Geometry: final body of the model. Coordinates: model frame, mm. A direction names the side the tool comes from. Give positions to 0.01 mm unless a question says otherwise; leave off trailing zeros. Loops run counter-clockwise (first coordinate to the right, second up) from the corner with the lowest first, then second, coordinate; pieces in that order, holes last.
from build123d import *

# Parameters (mm, degrees)
BOSS_EXTRUDE1_DEPTH      = 7
BOSS_EXTRUDE1_DEPTH_BACK = 7
BOSS_EXTRUDE2_DEPTH      = 7
BOSS_EXTRUDE3_DEPTH      = 7


with BuildPart() as part:
    # Sketch1 → Boss-Extrude1 (new, two sides: drawn at the far end of the back side and taken through both)
    with BuildSketch(Plane.XY.offset(-BOSS_EXTRUDE1_DEPTH_BACK)):
        with BuildLine():
            Line((-17.458418155, -11.36484808), (2.465475807, -9.621733225))
            ThreePointArc((2.465475807, -9.621733225), (6.955793602, -11.676837129), (7.491085956, -16.585998774))
            Line((7.491085956, -16.585998774), (-3.072780906, -41.033415882))
            ThreePointArc((-3.072780906, -41.033415882), (-2.24972743, -50.492456592), (6.106881965, -55))
            Line((6.106881965, -55), (21.106881965, -55))
            Line((21.106881965, -55), (21.106881965, -58))
            Line((21.106881965, -58), (6.106881965, -58))
            ThreePointArc((6.106881965, -58), (-3.921049309, -52.59094791), (-4.908713481, -41.240099059))
            Line((-4.908713481, -41.240099059), (5.655153382, -16.79268195))
            ThreePointArc((5.655153382, -16.79268195), (5.333977969, -13.847184963), (2.639787292, -12.614122621))
            Line((2.639787292, -12.614122621), (-17.197282581, -14.349641352))
            Line((-17.197282581, -14.349641352), (-17.458418155, -11.36484808))
        make_face()
    extrude(amount=BOSS_EXTRUDE1_DEPTH + BOSS_EXTRUDE1_DEPTH_BACK)

    # Sketch3 → Boss-Extrude2 (add)
    with BuildSketch(Plane.XY):
        with BuildLine():
            Line((2.465475807, -9.621733225), (26.965836734, -7.478229391))
            ThreePointArc((26.965836734, -7.478229391), (28.585544777, -8.088291477), (29.122784537, -9.733588816))
            Line((29.122784537, -9.733588816), (22.720894567, -58))
            Line((22.720894567, -58), (21.106881965, -58))
            Line((21.106881965, -58), (21.106881965, -55))
            Line((21.106881965, -55), (21.504791597, -55))
            Line((21.504791597, -55), (26.921714347, -14.159650971))
            ThreePointArc((26.921714347, -14.159650971), (26.115854708, -11.691704962), (23.686292644, -10.776611833))
            Line((23.686292644, -10.776611833), (2.726943035, -12.610317319))
            Line((2.726943035, -12.610317319), (2.465475807, -9.621733225))
        make_face()
    extrude(amount=BOSS_EXTRUDE2_DEPTH)

    # Sketch4 → Boss-Extrude3 (add)
    with BuildSketch(Plane.XY):
        Polygon((-15.197282581, -14.174664025), (-3.7781853, -38.623775477), (-2.92955004, -36.659822272), (-13.500697735, -14.026232084), align=None)
    extrude(amount=-BOSS_EXTRUDE3_DEPTH)


solid = part.part
Item 1: Section query D-D on y = -18.5. Return loops of the section in (x, z).
Values follow:
outline: (-13.18, -7) - (-11.41, -7) - (-11.41, 0) - (-13.18, 0) - close; (4.92, -7) - (6.66, -7) - (6.66, 7) - (4.92, 7) - close; (26.35, 0) - (27.96, 0) - (27.96, 7) - (26.35, 7) - close
Item 2: Set-up query: faces 4 (the face through (26, -23, 0)), 5 (the face through (21.107, -56, -4)), 6 (the face through (24.175, -34.866, 3.451)). Return all of +Z, -Z, +X, -X, +Y, -Y with unobstructed straight access to the full face (end or side cutting, diameter ignored); none if empty.
Values follow:
face 4: -Z, +X, +Y
face 5: -Z, +X, +Y, -Y
face 6: +Z, -Z
Item 3: Ray query, probe 1 along Z at (x, y) = (24, -47); probe 2 along Y at (x, z) = (5, 5); probe 3 along Y at (x, z) = (2, -5.25). Return the intervals inside material, ascending.
Values follow:
probe 1: z = 0 to 7
probe 2: y = -57.95 to -54.94, -22.35 to -18.31, -13.46 to -9.4
probe 3: y = -57.28 to -54.12, -29.29 to -25.25, -12.67 to -9.66
Item 4: Pin query (flat end, axial travel): pin 1 (3.5 mm diameter, centred on y = -57, z = -3.5, fed in from +X); pin 2 (7 mm diameter, centred on x = 12, z = 3, fed in from +Y); pin 3 (1.5 mm diameter, centred on x = -7, z = 3.5, fed in from +Y). Return the tip coordinate at first contact, or that it passes through.
Values follow:
pin 1: stops at x = 21.11
pin 2: stops at y = -8.48
pin 3: stops at y = -10.38
Item 5: Section query A-A on z = -1.25. Return loops of the section in (x, y), plus the area to 3 significant figures.
Values follow:
outline: (-17.46, -11.36) - (-17.2, -14.35) - (-15.2, -14.17) - (-3.78, -38.62) - (-4.91, -41.24) arc R12 ccw to (6.11, -58) - (21.11, -58) - (21.11, -55) - (6.11, -55) arc R10 cw to (-3.07, -41.03) - (7.49, -16.59) arc R5 ccw to (2.47, -9.62) - close; hole (-13.5, -14.03) - (-2.93, -36.66) - (5.66, -16.79) arc R3 ccw to (2.64, -12.61) - close
area: 263 mm2
Item 6: Section query B-B on y = -46.5. Return loops of the section in (x, z), plus the area to 3 significant figures.
Values follow:
outline: (-5.88, -7) - (-3.78, -7) - (-3.78, 7) - (-5.88, 7) - close; (22.63, 0) - (24.25, 0) - (24.25, 7) - (22.63, 7) - close
area: 40.7 mm2
Item 7: Draft query along Y for faces 1 (the face through (2.3, -28.6, -0.1)), 2 (the face through (0, -32, -7)), 3 (the face through (25.967, -33.529, 3.451)). Return one class per face: +Y half, -Y half, draft (parallel to the pull), parting line (faces both ways), or undercut.
Values follow:
face 1: undercut
face 2: draft
face 3: -Y half
Item 8: Section query C-C on x = 4.5. Return loops of the section in (y, z).
Values follow:
outline: (-57.89, -7) - (-54.87, -7) - (-54.87, 7) - (-57.89, 7) - close; (-23.51, -7) - (-19.47, -7) - (-19.47, 7) - (-23.51, 7) - close; (-13.06, -7) - (-9.87, -7) - (-9.87, 0) - (-9.44, 0) - (-9.44, 7) - (-13.06, 7) - close
